The model under review builds one solid part; all positions refer to its coordinate system, in mm. Round coordinates to 2 decimals unless told otherwise and drop trailing zeros. Loops run counter-clockwise (first coordinate to the right, second up) from the corner with the lowest first, then second, coordinate; pieces in that order, holes last. Notation, with made-up numbers: M 49,11 L 68,11 A30 ccw 68,33 Z; hole C 18.25,13 d3. An arc over 180 degrees is marked long. Answer as a JSON object with one key per item and string values. Group by question number.
Item 1: Insertion check: P1, Ø1.5, axis at x = 8.5, z = -10, coming from the -Y side. The pin has a flat end and moves straight along its axis. Give the tip position at first contact, or say it passes through.
Item 2: Consider section B-B (y = 0.7). State how many separate pieces and enclosed holes the cut face has, and give its area (3 significant figures).
Item 3: Consider section C-C (x = 29.5). Give the boundary of the cut face in (y, z).
Item 4: Consider section A-A (x = 1). Give the boundary of the cut face in (y, z).
Item 5: To check wall thickness, follow line 1 (Z direction, x = -1, y = 0.9); line 2 (Z direction, x = -9.76, y = 0.8); line 3 (Z direction, x = -8.76, y = 0.8). State the ranges of each line that lie inside material, in increasing order.
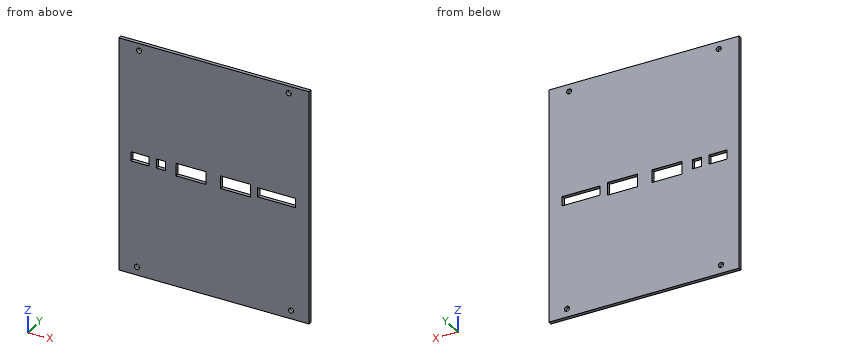
```python
from build123d import *

# Parameters (mm, degrees)
BOSS_EXTRUDE1_DEPTH            = 1.6
SKETCH3_W                      = 13
SKETCH3_H                      = 5.5
SKETCH3_W_2                    = 16.5
SKETCH3_H_2                    = 4
SKETCH3_W_3                    = 7.8
SKETCH3_W_4                    = 4
CUT_EXTRUDE2_DEPTH             = 49
F_2_2_2_2_DIAMETER_HOLE2_D     = 2.2
F_2_2_2_2_DIAMETER_HOLE2_DEPTH = 5
CUT_EXTRUDE4_REACH             = 3.6
SKETCH12_W                     = 83
SKETCH12_H                     = 2.5
SKETCH_1_W                     = 83
SKETCH_1_H                     = 1.6
EXTRUDE_1_DEPTH                = 1.6
SKETCH_2_W                     = 83
SKETCH_2_H                     = 1.6
EXTRUDE_2_DEPTH                = 1.6
F_2_2_2_2_DIAMETER_HOLE1_D     = 2.2
F_2_2_2_2_DIAMETER_HOLE1_DEPTH = 1.6
SKETCH16_W                     = 0.2
SKETCH16_H                     = 100.7
EXTRUDE1_DEPTH                 = 2.6


with BuildPart() as part:
    # Sketch1 → Boss-Extrude1 (new body)
    with BuildSketch(Plane(origin=(0, 0, 0), x_dir=(1, 0, 0), z_dir=(0, 1, 0))):
        Polygon((65.24, 0.272495156), (65.24, -46.437452638), (65.24, -63.637452638), (65.24, -70.137452638), (-17.76, -70.137452638), (-17.76, -63.637452638), (-17.76, -48.637452638), (-17.76, -45.78978272), (-17.76, 4.362547362), (-17.76, 21.562547362), (-17.76, 29.862547362), (65.24, 29.862547362), (65.24, 21.562547362), (65.24, 6.562547362), align=None)
    extrude(amount=BOSS_EXTRUDE1_DEPTH)

    # Sketch3 → Cut-Extrude2 (cut)
    with BuildSketch(Plane(origin=(0, 1.6, 0), x_dir=(1, 0, 0), z_dir=(0, 1, 0))):
        with Locations((13.74, -19.137452638)):
            Rectangle(SKETCH3_W, SKETCH3_H)
        with Locations((50.99, -19.337452638)):
            Rectangle(SKETCH3_W_2, SKETCH3_H_2)
        with Locations((-8.46, -19.337452638)):
            Rectangle(SKETCH3_W_3, SKETCH3_H_2)
        with Locations((33.04, -19.137452638)):
            Rectangle(SKETCH3_W, SKETCH3_H)
        with Locations((0.74, -19.337452638)):
            Rectangle(SKETCH3_W_4, SKETCH3_H_2)
    extrude(amount=-CUT_EXTRUDE2_DEPTH, mode=Mode.SUBTRACT)

    # Ø2.2 (2.2) Diameter Hole2
    with Locations(Plane(origin=(0, 1.6, 0), x_dir=(1, 0, 0), z_dir=(0, 1, 0))):
        with Locations((56.24, -66.137452638), (-8.76, -66.137452638)):
            Hole(F_2_2_2_2_DIAMETER_HOLE2_D / 2, depth=F_2_2_2_2_DIAMETER_HOLE2_DEPTH)

    # Sketch12 → Cut-Extrude4 (cut, up to next)
    with BuildSketch(Plane(origin=(0, 1.6, 0), x_dir=(1, 0, 0), z_dir=(0, 1, 0)), mode=Mode.PRIVATE) as cut_extrude4_sk1:
        with Locations((23.74, -68.887452638)):
            Rectangle(SKETCH12_W, SKETCH12_H)
    cut_extrude4_tool1 = extrude(cut_extrude4_sk1.sketch, amount=-CUT_EXTRUDE4_REACH, mode=Mode.PRIVATE) & part.part
    add(cut_extrude4_tool1.solids().sort_by_distance((23.74, 1.6, 68.887453))[0], mode=Mode.SUBTRACT)

    # ｽｹｯﾁ1 → ﾎﾞｽ - 押し出し1 (add)
    with BuildSketch(Plane(origin=(0, 0, -29.862547362), x_dir=(-1, 0, 0), z_dir=(0, 0, -1))):
        with Locations((-23.74, 0.8)):
            Rectangle(SKETCH_1_W, SKETCH_1_H)
    extrude(amount=EXTRUDE_1_DEPTH)

    # ｽｹｯﾁ2 → ﾎﾞｽ - 押し出し2 (add)
    with BuildSketch(Plane.XY.offset(67.637452638)):
        with Locations((23.74, 0.8)):
            Rectangle(SKETCH_2_W, SKETCH_2_H)
    extrude(amount=EXTRUDE_2_DEPTH)

    # Ø2.2 (2.2) Diameter Hole1
    with Locations(Plane(origin=(0, 1.6, 0), x_dir=(1, 0, 0), z_dir=(0, 1, 0))):
        with Locations((-9.76, 27.862547362), (57.24, 27.862547362)):
            Hole(F_2_2_2_2_DIAMETER_HOLE1_D / 2, depth=F_2_2_2_2_DIAMETER_HOLE1_DEPTH)

    # Sketch16 → Extrude1 (cut, through all)
    with BuildSketch(Plane(origin=(0, 1.6, 0), x_dir=(1, 0, 0), z_dir=(0, 1, 0))):
        with Locations((-17.66, -18.887452638)):
            Rectangle(SKETCH16_W, SKETCH16_H)
        with Locations((65.14, -18.887452638)):
            Rectangle(SKETCH16_W, SKETCH16_H)
    extrude(amount=-EXTRUDE1_DEPTH, mode=Mode.SUBTRACT)


solid = part.part
```
Geometry results:
{
 "1": {"P1": "stops at y = 0"},
 "2": {"separate pieces": "1", "enclosed holes": "9", "area": "8,050 mm^2"},
 "3": {"outline": "M 0,-31.46 L 1.6,-31.46 L 1.6,16.39 L 0,16.39 Z; M 0,21.89 L 1.6,21.89 L 1.6,69.24 L 0,69.24 Z"},
 "4": {"outline": "M 0,-31.46 L 1.6,-31.46 L 1.6,17.34 L 0,17.34 Z; M 0,21.34 L 1.6,21.34 L 1.6,69.24 L 0,69.24 Z"},
 "5": {"line 1": "z = -31.46 to 17.34, 21.34 to 69.24", "line 2": "z = -31.46 to -28.96, -26.76 to 17.34, 21.34 to 65.68, 66.6 to 69.24", "line 3": "z = -31.46 to -28.32, -27.4 to 17.34, 21.34 to 65.04, 67.24 to 69.24"}
}
